```python
from build123d import *

# Parameters (mm, degrees)
F0_R            = 8
F1_DEPTH        = 40
F2_W            = 37
F2_H            = 37
F3_DEPTH        = 1.5
F3_COPIES_COUNT = 5
F4_SIZE         = 1.49999
F5_R            = 3
F6_DEPTH        = 20
F7_R            = 2
F8_T1_DEPTH     = 37.093829888
F8_T3_DEPTH     = 37.093829888
F8_T5_DEPTH     = 37.093829888
F8_T7_DEPTH     = 37.093829888
F8_T9_DEPTH     = 37.093829888
F8_T12_ANGLE    = 72
F8_T14_ANGLE    = 72
F8_T16_ANGLE    = 72
F8_T18_ANGLE    = 72
F8_T20_ANGLE    = 72
F8_T22_ANGLE    = 72
F8_T24_ANGLE    = 72
F8_T26_ANGLE    = 72
F8_T28_ANGLE    = 72
F8_T30_ANGLE    = 72
F9_R            = 1.5
F10_DEPTH       = 10


# Not quite as in the source:
# - a fillet or chamfer that OpenCascade refuses, or shapes differently, is made with other operations: its cross-section is extruded or revolved along the edge and cut away or added
# - a fillet or chamfer is up to 0.001 mm smaller than in the source, because OpenCascade refuses the exact size
# - a pattern or mirror of a feature is missing from the dataset's text; its kind, count and spacing are read off the source's solid


with BuildPart() as f1:
    # F0 (on Top) → F1 (new body)
    with BuildSketch(Plane.XY):
        Polygon((27.5276384094, -20), (27.5276384094, 20), (-10.5146222424, 32.360679775), (-34.0260323341, 0), (-10.5146222424, -32.360679775), align=None)
        Circle(F0_R, mode=Mode.SUBTRACT)
    extrude(amount=F1_DEPTH)

    # F2 (on face) → F3 (cut)
    with BuildSketch(Plane.YZ.offset(27.5276384094)):
        with Locations((0, 20)):
            Rectangle(F2_W, F2_H)
    f3 = extrude(amount=-F3_DEPTH, mode=Mode.SUBTRACT)

    # F3_copies: F3 ×5 about axis
    f3_copies_axis = Axis((0, 0, 0), (0, 0, 1))
    for i in range(1, F3_COPIES_COUNT):
        add(f3.rotate(f3_copies_axis, i * 360 / F3_COPIES_COUNT), mode=Mode.SUBTRACT)

    # F4 (size 1.5 in the source; OpenCascade refuses exactly that, so slightly less here)
    f4_edges = [f1.edges().sort_by_distance(p)[0] for p in [
        (26.027638, 0, 38.5),
        (26.027638, -18.5, 20),
        (26.027638, 0, 1.5),
        (26.027638, 18.5, 20),
        (25.637528, -19.036941, 20),
        (8.042983, -24.753755, 1.5),
        (-9.551563, -30.47057, 20),
        (8.042983, -24.753755, 38.5),
        (-9.551563, 30.47057, 20),
        (8.042983, 24.753755, 1.5),
        (25.637528, 19.036941, 20),
        (8.042983, 24.753755, 38.5),
        (-10.182775, -30.265476, 20),
        (-21.056802, -15.298662, 1.5),
        (-31.930829, -0.331848, 20),
        (-21.056802, -15.298662, 38.5),
        (-31.930829, 0.331848, 20),
        (-21.056802, 15.298662, 1.5),
        (-10.182775, 30.265476, 20),
        (-21.056802, 15.298662, 38.5),
    ]]
    chamfer(f4_edges, length=F4_SIZE)

    # F5 (on Right) → F6 (cut)
    with BuildSketch(Plane.YZ):
        with Locations((0, 49.5)):
            Circle(F5_R)
    extrude(amount=F6_DEPTH, mode=Mode.SUBTRACT)

    # F7
    f7_edges = [f1.edges().sort_by_distance(p)[0] for p in [
        (-34.026032, 0, 20),
        (-10.514622, -32.36068, 20),
        (27.527638, -20, 20),
        (27.527638, 20, 20),
        (-10.514622, 32.36068, 20),
    ]]
    fillet(f7_edges, radius=F7_R)

    # F8: fillet of radius 2 on 12 edges, made by hand

    # F8_s2 → F8_t1 (cut)
    with BuildSketch(Plane(origin=(-17.6391643147, -5.7313119109, 0), x_dir=(0, 0, 1), z_dir=(0.9510565163, 0.3090169944, 0))):
        with BuildLine():
            ThreePointArc((40, 25.5276384094), (39.4142135624, 26.9418519718), (38, 27.5276384094))
            Line((38, 27.5276384094), (40, 27.5276384094))
            Line((40, 27.5276384094), (40, 25.5276384094))
        make_face()
        with BuildLine():
            ThreePointArc((0, 25.5276384094), (0.5857864376, 26.9418519718), (2, 27.5276384094))
            Line((2, 27.5276384094), (0, 27.5276384094))
            Line((0, 27.5276384094), (0, 25.5276384094))
        make_face()
    extrude(amount=F8_T1_DEPTH, mode=Mode.SUBTRACT)

    # F8_s4 → F8_t3 (cut)
    with BuildSketch(Plane(origin=(-10.9016030796, 15.0047693829, 0), x_dir=(0, 0, 1), z_dir=(0.5877852523, -0.8090169944, 0))):
        with BuildLine():
            ThreePointArc((40, 25.5276384094), (39.4142135624, 26.9418519718), (38, 27.5276384094))
            Line((38, 27.5276384094), (40, 27.5276384094))
            Line((40, 27.5276384094), (40, 25.5276384094))
        make_face()
        with BuildLine():
            ThreePointArc((0, 25.5276384094), (0.5857864376, 26.9418519718), (2, 27.5276384094))
            Line((2, 27.5276384094), (0, 27.5276384094))
            Line((0, 27.5276384094), (0, 25.5276384094))
        make_face()
    extrude(amount=F8_T3_DEPTH, mode=Mode.SUBTRACT)

    # F8_s6 → F8_t5 (cut)
    with BuildSketch(Plane(origin=(10.9016030796, 15.0047693829, 0), x_dir=(0, 0, 1), z_dir=(-0.5877852523, -0.8090169944, 0))):
        with BuildLine():
            ThreePointArc((40, 25.5276384094), (39.4142135624, 26.9418519718), (38, 27.5276384094))
            Line((38, 27.5276384094), (40, 27.5276384094))
            Line((40, 27.5276384094), (40, 25.5276384094))
        make_face()
        with BuildLine():
            ThreePointArc((0, 25.5276384094), (0.5857864376, 26.9418519718), (2, 27.5276384094))
            Line((2, 27.5276384094), (0, 27.5276384094))
            Line((0, 27.5276384094), (0, 25.5276384094))
        make_face()
    extrude(amount=F8_T5_DEPTH, mode=Mode.SUBTRACT)

    # F8_s8 → F8_t7 (cut)
    with BuildSketch(Plane(origin=(17.6391643147, -5.7313119109, 0), x_dir=(0, 0, 1), z_dir=(-0.9510565163, 0.3090169944, 0))):
        with BuildLine():
            ThreePointArc((40, 25.5276384094), (39.4142135624, 26.9418519718), (38, 27.5276384094))
            Line((38, 27.5276384094), (40, 27.5276384094))
            Line((40, 27.5276384094), (40, 25.5276384094))
        make_face()
        with BuildLine():
            ThreePointArc((0, 25.5276384094), (0.5857864376, 26.9418519718), (2, 27.5276384094))
            Line((2, 27.5276384094), (0, 27.5276384094))
            Line((0, 27.5276384094), (0, 25.5276384094))
        make_face()
    extrude(amount=F8_T7_DEPTH, mode=Mode.SUBTRACT)

    # F8_s10 → F8_t9 (cut)
    with BuildSketch(Plane.XZ.offset(-18.546914944)):
        with BuildLine():
            ThreePointArc((27.5276384094, 38), (26.9418519718, 39.4142135624), (25.5276384094, 40))
            Line((25.5276384094, 40), (27.5276384094, 40))
            Line((27.5276384094, 40), (27.5276384094, 38))
        make_face()
        with BuildLine():
            ThreePointArc((27.5276384094, 2), (26.9418519718, 0.5857864376), (25.5276384094, 0))
            Line((25.5276384094, 0), (27.5276384094, 0))
            Line((27.5276384094, 0), (27.5276384094, 2))
        make_face()
    extrude(amount=F8_T9_DEPTH, mode=Mode.SUBTRACT)

    # F8_s11 → F8_t12 (revolve, cut)
    with BuildSketch(Plane.XZ.offset(18.546914944)):
        with BuildLine():
            ThreePointArc((25.5276384094, 0), (26.9418519718, 0.5857864376), (27.5276384094, 2))
            Line((27.5276384094, 2), (27.5276384094, 0))
            Line((27.5276384094, 0), (25.5276384094, 0))
        make_face()
    revolve(axis=Axis((25.5276384094, -18.546914944, 0), (0, 0, -1)), revolution_arc=F8_T12_ANGLE, mode=Mode.SUBTRACT)

    # F8_s13 → F8_t14 (revolve, cut)
    with BuildSketch(Plane.XZ.offset(-18.546914944)):
        with BuildLine():
            ThreePointArc((25.5276384094, 0), (26.9418519718, 0.5857864376), (27.5276384094, 2))
            Line((27.5276384094, 2), (27.5276384094, 0))
            Line((27.5276384094, 0), (25.5276384094, 0))
        make_face()
    revolve(axis=Axis((25.5276384094, 18.546914944, 0), (0, 0, 1)), revolution_arc=F8_T14_ANGLE, mode=Mode.SUBTRACT)

    # F8_s15 → F8_t16 (revolve, cut)
    with BuildSketch(Plane(origin=(-17.6391643147, -5.7313119109, 0), x_dir=(0, 0, 1), z_dir=(0.9510565163, 0.3090169944, 0))):
        with BuildLine():
            ThreePointArc((0, 25.5276384094), (0.5857864376, 26.9418519718), (2, 27.5276384094))
            Line((2, 27.5276384094), (0, 27.5276384094))
            Line((0, 27.5276384094), (0, 25.5276384094))
        make_face()
    revolve(axis=Axis((-9.7506902199, -30.0095387658, 0), (0, 0, -1)), revolution_arc=F8_T16_ANGLE, mode=Mode.SUBTRACT)

    # F8_s17 → F8_t18 (revolve, cut)
    with BuildSketch(Plane(origin=(-17.6391643147, 5.7313119109, 0), x_dir=(0, 0, 1), z_dir=(0.9510565163, -0.3090169944, 0))):
        with BuildLine():
            ThreePointArc((0, -25.5276384094), (0.5857864376, -26.9418519718), (2, -27.5276384094))
            Line((2, -27.5276384094), (0, -27.5276384094))
            Line((0, -27.5276384094), (0, -25.5276384094))
        make_face()
    revolve(axis=Axis((-9.7506902199, 30.0095387658, 0), (0, 0, 1)), revolution_arc=F8_T18_ANGLE, mode=Mode.SUBTRACT)

    # F8_s19 → F8_t20 (revolve, cut)
    with BuildSketch(Plane(origin=(-10.9016030796, 15.0047693829, 0), x_dir=(0, 0, 1), z_dir=(0.5877852523, -0.8090169944, 0))):
        with BuildLine():
            ThreePointArc((0, 25.5276384094), (0.5857864376, 26.9418519718), (2, 27.5276384094))
            Line((2, 27.5276384094), (0, 27.5276384094))
            Line((0, 27.5276384094), (0, 25.5276384094))
        make_face()
    revolve(axis=Axis((-31.5538963791, 0, 0), (0, 0, -1)), revolution_arc=F8_T20_ANGLE, mode=Mode.SUBTRACT)

    # F8_s21 → F8_t22 (revolve, cut)
    with BuildSketch(Plane.XZ.offset(18.546914944)):
        with BuildLine():
            ThreePointArc((27.5276384094, 38), (26.9418519718, 39.4142135624), (25.5276384094, 40))
            Line((25.5276384094, 40), (27.5276384094, 40))
            Line((27.5276384094, 40), (27.5276384094, 38))
        make_face()
    revolve(axis=Axis((25.5276384094, -18.546914944, 40), (0, 0, -1)), revolution_arc=F8_T22_ANGLE, mode=Mode.SUBTRACT)

    # F8_s23 → F8_t24 (revolve, cut)
    with BuildSketch(Plane.XZ.offset(-18.546914944)):
        with BuildLine():
            ThreePointArc((27.5276384094, 38), (26.9418519718, 39.4142135624), (25.5276384094, 40))
            Line((25.5276384094, 40), (27.5276384094, 40))
            Line((27.5276384094, 40), (27.5276384094, 38))
        make_face()
    revolve(axis=Axis((25.5276384094, 18.546914944, 40), (0, 0, 1)), revolution_arc=F8_T24_ANGLE, mode=Mode.SUBTRACT)

    # F8_s25 → F8_t26 (revolve, cut)
    with BuildSketch(Plane(origin=(-17.6391643147, -5.7313119109, 0), x_dir=(0, 0, 1), z_dir=(0.9510565163, 0.3090169944, 0))):
        with BuildLine():
            ThreePointArc((40, 25.5276384094), (39.4142135624, 26.9418519718), (38, 27.5276384094))
            Line((38, 27.5276384094), (40, 27.5276384094))
            Line((40, 27.5276384094), (40, 25.5276384094))
        make_face()
    revolve(axis=Axis((-9.7506902199, -30.0095387658, 40), (0, 0, -1)), revolution_arc=F8_T26_ANGLE, mode=Mode.SUBTRACT)

    # F8_s27 → F8_t28 (revolve, cut)
    with BuildSketch(Plane(origin=(-17.6391643147, 5.7313119109, 0), x_dir=(0, 0, 1), z_dir=(0.9510565163, -0.3090169944, 0))):
        with BuildLine():
            ThreePointArc((40, -25.5276384094), (39.4142135624, -26.9418519718), (38, -27.5276384094))
            Line((38, -27.5276384094), (40, -27.5276384094))
            Line((40, -27.5276384094), (40, -25.5276384094))
        make_face()
    revolve(axis=Axis((-9.7506902199, 30.0095387658, 40), (0, 0, 1)), revolution_arc=F8_T28_ANGLE, mode=Mode.SUBTRACT)

    # F8_s29 → F8_t30 (revolve, cut)
    with BuildSketch(Plane(origin=(-10.9016030796, 15.0047693829, 0), x_dir=(0, 0, 1), z_dir=(0.5877852523, -0.8090169944, 0))):
        with BuildLine():
            ThreePointArc((40, 25.5276384094), (39.4142135624, 26.9418519718), (38, 27.5276384094))
            Line((38, 27.5276384094), (40, 27.5276384094))
            Line((40, 27.5276384094), (40, 25.5276384094))
        make_face()
    revolve(axis=Axis((-31.5538963791, 0, 40), (0, 0, -1)), revolution_arc=F8_T30_ANGLE, mode=Mode.SUBTRACT)

    # F9 (on Right) → F10 (cut)
    with BuildSketch(Plane.YZ):
        with Locations((0, 20)):
            Circle(F9_R)
    extrude(amount=F10_DEPTH, mode=Mode.SUBTRACT)


solid = f1.part
```
Geometry check sheet. Reference: the model listing, model coordinates, mm. A direction names the side the tool comes from. Give positions to 0.01 mm unless a question says otherwise; leave off trailing zeros. One line per question, with ' | ' between items.
Item 1: Access from +Z, -Z, +X, -X, +Y, -Y to the whole of each face (thin tool, end or side, straight path). Record for faces 5 (the flat face through (-8.6, -30.94, 19.74)), 6 (the cylindrical face through (8.484, 25.272, 39.651)), 7 (the cylindrical face through (26.957, 0.26, 39.399)), 8 (the flat face through (26.77, -17.74, 19.74)), 9 (the flat face through (-11.228, 30.085, 19.742)).
Determined:
face 5: +X, -Y | face 6: +Z, +X, +Y | face 7: +Z, +X, +Y, -Y | face 8: +X | face 9: -X
Item 2: Draft check along X on faces 1 (the flat face through (10, 0, 20)), 2 (the cylindrical face through (-21.63, 16.04, 0.57)), 3 (the cylindrical face through (27.156, 19.708, 20.252)), 4 (the cylindrical face through (-1.73, -7.81, 19.72)). Enter one of: released by +X, released by -X, zero draft, split by the parting line, or undercut.
Determined:
face 1: undercut | face 2: released by -X | face 3: released by +X | face 4: undercut
Item 3: Scan lines: line 1 along Z through (x, y) = (8.6, 0); line 2 along Y through (x, z) = (9.25, 20); line 3 along Z through (x, y) = (-18.5, 19). Record each from-to range of solid material in increasing order.
Determined:
line 1: 0 to 18.5, 21.5 to 40 | line 2: -24.36 to -1.5, 1.5 to 24.36 | line 3: 0.09 to 2.89, 37.11 to 39.91
Item 4: Depth check by flat-ended pin: pin 1 (6 mm diameter, centred on y = 15.5, z = 13, fed in from -X); pin 2 (1.5 mm diameter, centred on x = 16, z = 16.5, fed in from +Y); pin 3 (3 mm diameter, centred on y = -21, z = 12, fed in from -X). Enter the tip coordinate at first touch or a pass-through.
Determined:
pin 1: x = -23.09 | pin 2: y = 22.41 | pin 3: x = -18
